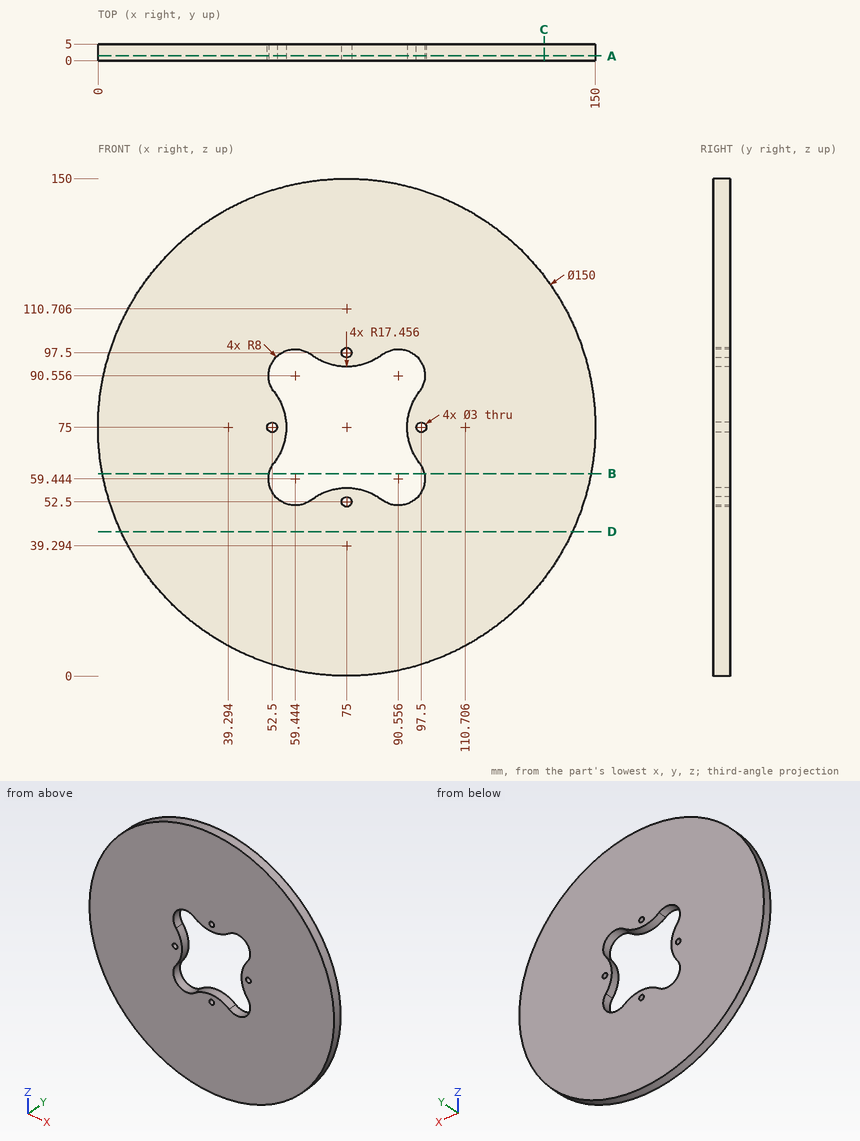
Verification items for this drawing (mm, ordinates from the low corner). Give positions to 0.01 mm unless a question says otherwise; leave off trailing zeros. Order: outer loops, then holes, each group sorted by start corner. A loop starts at its lowest first (then second) coordinate and runs counter-clockwise, first axis right, second up.
1) Material ranges on probe 1 along Z at (x, y) = (52.5, 3.6) (1 decimal); probe 2 along Z at (x, y) = (53, 2.8) (1 decimal); probe 3 along X at (y, z) = (2.1, 85), recorded low to high.
Results are:
probe 1: z = 3.5 to 55.5, 63.4 to 73.5, 76.5 to 86.6, 94.5 to 146.5
probe 2: z = 3.3 to 54.7, 64.2 to 73.6, 76.4 to 85.8, 95.3 to 146.7
probe 3: x = 0.67 to 53.6, 96.4 to 149.33
2) Gauge pin test, flat ends, axial feed: pin 1 (2 mm diameter, centred on x = 92.5, z = 20.5, fed in from -Y); pin 2 (1 mm diameter, centred on x = 96.5, y = 1, fed in from -Z). Record the tip position at first contact, or that the pin passes through.
Results are:
pin 1: stops at y = 0
pin 2: stops at z = 3
3) Cross-section at D-D (z = 43.5). Record the boundary of the cut face in (x, y).
Results are:
outline: (6.94, 0) - (143.06, 0) - (143.06, 5) - (6.94, 5) - close
4) Cross-section at B-B (z = 61). Record the boundary of the cut face in (x, y), then the cut area to 3 significant figures.
Results are:
outline: (1.32, 0) - (51.6, 0) - (51.6, 5) - (1.32, 5) - close; (98.4, 0) - (148.68, 0) - (148.68, 5) - (98.4, 5) - close
area: 503 mm2
5) Cross-section at C-C (x = 134.5). Record the boundary of the cut face in (y, z).
Results are:
outline: (0, 29.34) - (5, 29.34) - (5, 120.66) - (0, 120.66) - close
6) Cross-section at A-A (y = 1.4). Record the boundary of the cut face in (x, z), then the cut area to 3 significant figures.
Results are:
outline: circle Ø150 at (75, 75); hole circle Ø3 at (52.5, 75); hole (53.11, 64.33) arc R8 ccw to (64.33, 53.11) arc R17.46 cw to (85.67, 53.11) arc R8 ccw to (96.89, 64.33) arc R17.46 cw to (96.89, 85.67) arc R8 ccw to (85.67, 96.89) arc R17.46 cw to (64.33, 96.89) arc R8 ccw to (53.11, 85.67) arc R17.46 cw to start; hole circle Ø3 at (75, 52.5); hole circle Ø3 at (75, 97.5); hole circle Ø3 at (97.5, 75)
area: 15,900 mm2
